CAD build for the part. Positions are in the model's coordinates, mm. A direction names the side the tool comes from. Give positions to 0.01 mm unless a question says otherwise; leave off trailing zeros. Loops run counter-clockwise (first coordinate to the right, second up) from the corner with the lowest first, then second, coordinate; pieces in that order, holes last. Notation, with made-up numbers: (73.25, 40.5) -> (84.25, 40.5) arc R23 ccw to (84.25, 78.5) -> close; hole circle Ø3 at (-4.75, 16.25). An arc over 180 degrees is marked (long way). Write each question's results on one line, items separated by ' | '. Start each with the question number.
```python
from build123d import *

# Parameters (mm, degrees)
F0_W     = 19
F0_H     = 24
F1_DEPTH = 4
F3_DEPTH = 19
F4_W     = 2
F4_H     = 10.4102807478
F7_DEPTH = 24.001


with BuildPart() as f1:
    # F0 (on Right) → F1 (new body)
    with BuildSketch(Plane.YZ):
        Rectangle(F0_W, F0_H)
    extrude(amount=F1_DEPTH)

    # F2 (on face) → F3 (join, through all)
    with BuildSketch(Plane(origin=(0, 9.5, 0), x_dir=(-1, 0, 0), z_dir=(0, 1, 0))):
        with BuildLine():
            Line((2, 6), (0, 6))
            Line((0, 6), (0, -15.05894568))
            ThreePointArc((0, -15.05894568), (1.4823619098, -16.9907973326), (3.7320508076, -16.05894568))
            Line((3.7320508076, -16.05894568), (14.6008684854, 2.7663987562))
            Line((14.6008684854, 2.7663987562), (12.4102807478, 4.0311351762))
            Line((12.4102807478, 4.0311351762), (2, -14))
            Line((2, -14), (2, 6))
        make_face()
    extrude(amount=-F3_DEPTH)

    # F4 (on face) → F5 (join, up to the next surface of F1)
    with BuildSketch(Plane(origin=(-7.5621778265, 0, -4.3660254038), x_dir=(0, 1, 0), z_dir=(0.8660254038, 0, 0.5))):
        with Locations((0, -5.9192152791)):
            Rectangle(F4_W, F4_H)
    extrude(until=Until.NEXT)

    # F6 (on face) → F7 (cut, through all)
    with BuildSketch(Plane(origin=(0, 0, -12), x_dir=(1, 0, 0), z_dir=(0, 0, -1))):
        with BuildLine():
            Line((4, -7.5), (4, 7.5))
            ThreePointArc((4, 7.5), (0.9658907755, 0), (4, -7.5))
        make_face()
    extrude(amount=-F7_DEPTH, mode=Mode.SUBTRACT)


solid = f1.part
```
Q1. Drop flat-ended pins along their axis: pin 1 (5 mm diameter, centred on y = 1, z = -10, fed in from -X); pin 2 (1 mm diameter, centred on y = -1, z = -4.5, fed in from -X); pin 3 (5 mm diameter, centred on y = -2, z = -3.5, fed in from +X); pin 4 (3 mm diameter, centred on x = -2.5, z = -4, fed in from +Y). Give the stop position or say it passes through.
Q2. Saw through at A-A, the plane y = 8. List the corners of the cut face in (x, z), then the cut area to 3 significant figures.
Q3. Saw through at D-D, the plane z = -9.5. List the corners of the cut face in (x, y), then the cut area to 3 significant figures.
Q4. Wall check: L1, parallel to Y at x = -2.5, z = -11.5; L2, parallel to X at y = 8.25, z = 3; L3, parallel to X at y = 4.75, z = -12.5. Give the ranges that are in metal, low to high.
Q5. Which spindle directions (+Z, -Z, +X, -X, +Y, -Y) get a long thin tool onto all of the face, cutting with end or side? Do faces 5 (the face through (-4, 1, -7)), 6 (the face through (-8.435, 0.133, -2.855)), 7 (the face through (0, 0, 9)), 8 (the face through (0, 0, -14)). Say none if no direction does.
Q6. Mould opens along X. For faces 1 (the face through (-2, 2, -4)), 2 (the face through (0.6, -0.1, -12)), 3 (the face through (-4, -1, -7)), 4 (the face through (-9.09, 0.13, -6.78)) say: pulls with the +X half, pulls with the -X half, needs draft (parallel to the pull), parting line crosses it, or undercut.
Q7. Saw through at C-C, the plane z = 1.5. List the corners of the cut face in (x, y).
Q8. Saw through at B-B, the plane x = 1.5. List the corners of the cut face in (y, z).
Answer block:
1) pin 1: stops at x = -8.67 | pin 2: stops at x = -10.69 | pin 3: stops at x = 1.95 | pin 4: stops at y = 9.5
2) outline: (-14.6, 2.77) -> (-3.73, -16.06) arc R2 ccw to (0, -15.06) -> (0, -12) -> (4, -12) -> (4, 12) -> (0, 12) -> (0, 6) -> (-2, 6) -> (-2, -14) -> (-12.41, 4.03) -> close | area: 198 mm2
3) outline: (-7.52, -9.5) -> (-4.6, -9.5) -> (-4.6, -1) -> (-2, -1) -> (-2, -9.5) -> (4, -9.5) -> (4, -7.5) arc R10.79 cw to (4, 7.5) -> (4, 9.5) -> (-2, 9.5) -> (-2, 1) -> (-4.6, 1) -> (-4.6, 9.5) -> (-7.52, 9.5) -> close | area: 143 mm2
4) L1: y = -1 to 1 | L2: x = -14.2 to -11.81, -2 to 4 | L3: x = -5.79 to -2.87, -2 to 0
5) face 5: +Z, +Y | face 6: +Z | face 7: +Z, -X, +Y, -Y | face 8: -Z, +X, +Y, -Y
6) face 1: undercut | face 2: needs draft | face 3: undercut | face 4: pulls with the -X half
7) outline: (-13.87, -9.5) -> (-10.95, -9.5) -> (-10.95, 9.5) -> (-13.87, 9.5) -> close; (-2, -9.5) -> (4, -9.5) -> (4, -7.5) arc R10.79 cw to (4, 7.5) -> (4, 9.5) -> (-2, 9.5) -> close
8) outline: (-9.5, -12) -> (-3.35, -12) -> (-3.35, 12) -> (-9.5, 12) -> close; (3.35, -12) -> (9.5, -12) -> (9.5, 12) -> (3.35, 12) -> close
